```python
from build123d import *

# Parameters (mm, degrees)
BOSS_EXTRUDE1_DEPTH = 6
SKETCH2_W           = 30
SKETCH2_H           = 14
SKETCH2_W_2         = 97
SKETCH2_H_2         = 40
SKETCH2_W_3         = 47
SKETCH2_H_3         = 57
CUT_EXTRUDE1_DEPTH  = 6


with BuildPart() as part:
    # Model → Boss-Extrude1 (new body)
    with BuildSketch(Plane.XY):
        Polygon((209, 406), (209, 384), (203, 384), (203, 372), (209, 372), (209, 360), (203, 360), (203, 348), (209, 348), (209, 336), (203, 336), (203, 324), (209, 324), (209, 312), (203, 312), (203, 300), (209, 300), (209, 288), (203, 288), (203, 276), (209, 276), (209, 264), (203, 264), (203, 252), (209, 252), (209, 240), (203, 240), (203, 228), (209, 228), (209, 216), (209, 206), (227, 206), (227, 212), (239, 212), (239, 206), (251, 206), (251, 212), (263, 212), (263, 206), (275, 206), (275, 212), (287, 212), (287, 206), (299, 206), (299, 212), (311, 212), (311, 206), (323, 206), (323, 212), (335, 212), (335, 206), (347, 206), (347, 212), (359, 212), (359, 206), (371, 206), (371, 212), (383, 212), (383, 206), (395, 206), (395, 212), (407, 212), (407, 206), (419, 206), (419, 212), (431, 212), (431, 206), (443, 206), (443, 212), (455, 212), (455, 206), (467, 206), (467, 212), (479, 212), (479, 206), (491, 206), (497, 206), (497, 228), (503, 228), (503, 240), (497, 240), (497, 252), (503, 252), (503, 264), (497, 264), (497, 276), (503, 276), (503, 288), (497, 288), (497, 300), (503, 300), (503, 312), (497, 312), (497, 324), (503, 324), (503, 336), (497, 336), (497, 348), (503, 348), (503, 360), (497, 360), (497, 372), (503, 372), (503, 384), (497, 384), (497, 396), (497, 406), (479, 406), (479, 400), (467, 400), (467, 406), (455, 406), (455, 400), (443, 400), (443, 406), (431, 406), (431, 400), (419, 400), (419, 406), (407, 406), (407, 400), (395, 400), (395, 406), (383, 406), (383, 400), (371, 400), (371, 406), (359, 406), (359, 400), (347, 400), (347, 406), (335, 406), (335, 400), (323, 400), (323, 406), (311, 406), (311, 400), (299, 400), (299, 406), (287, 406), (287, 400), (275, 400), (275, 406), (263, 406), (263, 400), (251, 400), (251, 406), (239, 406), (239, 400), (227, 400), (227, 406), (215, 406), align=None)
    extrude(amount=BOSS_EXTRUDE1_DEPTH)

    # Sketch2 → Cut-Extrude1 (cut)
    with BuildSketch(Plane.XY.offset(6)):
        with Locations((353, 375)):
            Rectangle(SKETCH2_W, SKETCH2_H)
        with Locations((353, 326)):
            Rectangle(SKETCH2_W_2, SKETCH2_H_2)
        with Locations((353, 260.5)):
            Rectangle(SKETCH2_W_3, SKETCH2_H_3)
    extrude(amount=-CUT_EXTRUDE1_DEPTH, mode=Mode.SUBTRACT)


solid = part.part
```
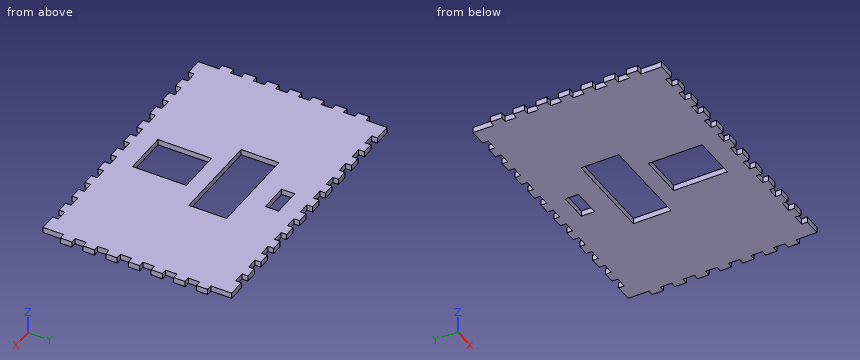
Input: part model. Units: mm. Frame: model coordinates. Round coordinates to 2 decimals unless told otherwise and drop trailing zeros. Loops run counter-clockwise (first coordinate to the right, second up) from the corner with the lowest first, then second, coordinate; pieces in that order, holes last. Notation, with made-up numbers: (32, -1) -> (54, -1) arc R27 cw to (54, 23) -> close; hole circle Ø4 at (41.5, 44.5). An arc over 180 degrees is marked (long way). Use one line per item in the form item = value. Start each with the question number.
Item 1: Section query A-A on x = 387. Return the cut outline in (y, z).
Item 2: Contact query for flat-ended pins moving along their axis: pin 1 Ø1.8 at (y, z) = (210, 2.5) entering from +X; pin 2 Ø3 at (x, z) = (308, 1.5) entering from +Y; pin 3 Ø1.5 at (x, z) = (251.5, 4.5) entering from -Y; pin 4 Ø3 at (x, z) = (376, 2) entering from -Y. Output: stop coordinate, or through.
Item 3: Section query D-D on y = 393.5. Return the cut outline in (x, z), then the cut area to 3 significant figures.
Item 4: Section query B-B on y = 282. Return the cut outline in (x, z), then the cut area to 3 significant figures.
Item 5: Section query C-C on z = 3.05. Count the separate pieces of the cut face and the enclosed holes in it, then the cut area to 3 significant figures.
Item 6: Material intervals for L1, parallel to X at y = 330, z = 2.45; L2, parallel to Y at x = 310, z = 5.7; L3, parallel to X at y = 313.5, z = 1.4, sorted ascending. Write a range as from..to.
Ans:
q1.outline = (206, 0) -> (306, 0) -> (306, 6) -> (206, 6) -> close; (346, 0) -> (406, 0) -> (406, 6) -> (346, 6) -> close
q2.pin_1 = 497
q2.pin_2 = 400
q2.pin_3 = 206
q2.pin_4 = 212
q3.outline = (209, 0) -> (497, 0) -> (497, 6) -> (209, 6) -> close
q3.area = 1,730 mm^2
q4.outline = (203, 0) -> (329.5, 0) -> (329.5, 6) -> (203, 6) -> close; (376.5, 0) -> (503, 0) -> (503, 6) -> (376.5, 6) -> close
q4.area = 1,520 mm^2
q5.separate_pieces = 1
q5.enclosed_holes = 3
q5.area = 50,000 mm^2
q6.L1 = 203..304.5, 401.5..503
q6.L2 = 212..306, 346..400
q6.L3 = 209..304.5, 401.5..497
